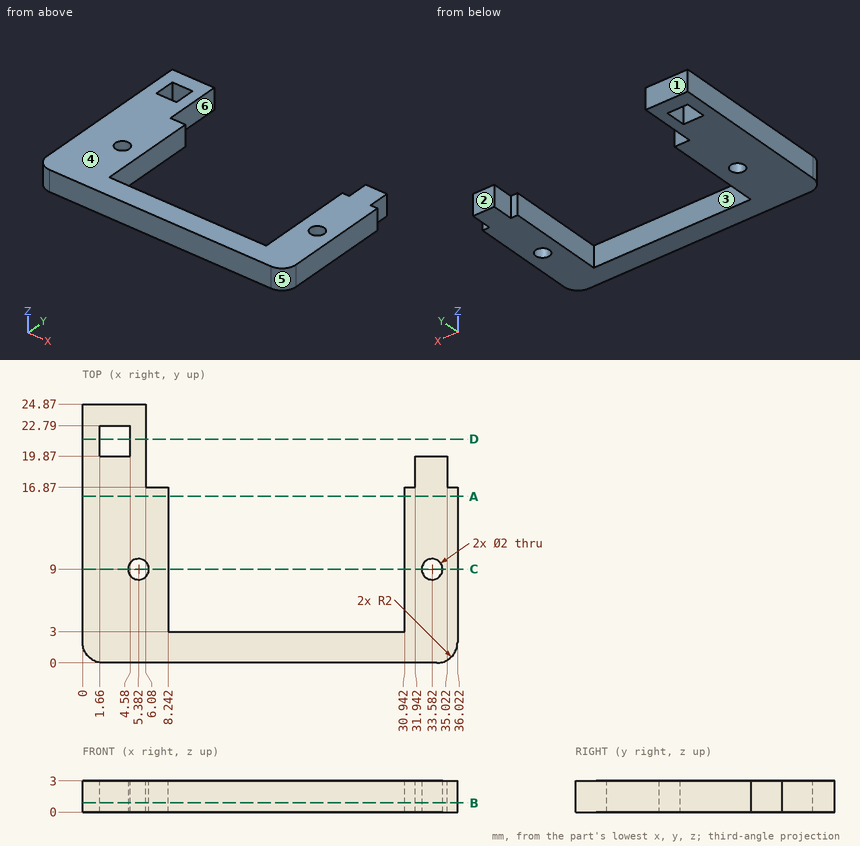
Input: dimensioned drawing with shaded views. Units: mm. Origin: part minimum x, y, z. A direction names the side the tool comes from. Round coordinates to 2 decimals unless told otherwise and drop trailing zeros. Loops run counter-clockwise (first coordinate to the right, second up) from the corner with the lowest first, then second, coordinate; pieces in that order, holes last. Notation, with made-up numbers: (0, 36.25) -> (44, 36.25) arc R13 ccw to (44, 60.25) -> close; hole circle Ø4 at (-24.5, 2.25). An arc over 180 degrees is marked (long way). Answer as a JSON object with one key per item and string values. Group by question number.
1) Section query B-B on z = 0.9. Output: boundary loops of the cut face in (x, y), plus the area to 3 significant figures.
2) Reachability of the marked faces 1, 2 and 3 from +Z, -Z, +X, -X, +Y, -Y: full face, straight path, thin tool, end or side. Return the list, or none.
3) Section query C-C on y = 9. Output: boundary loops of the cut face in (x, z).
4) Section query A-A on y = 16. Output: boundary loops of the cut face in (x, z).
5) Pin query (flat end, axial travel): pin 1 (1.5 mm diameter, centred on y = 20.5, z = 1, fed in from +X); pin 2 (1.5 mm diameter, centred on y = 21, z = 1.5, fed in from +X); pin 3 (0.6 mm diameter, centred on x = 7, z = 1, fed in from +Y). Return the tip coordinate at first contact, or that it passes through.
6) Ray query, L1, parallel to X at y = 14.5, z = 2.4; L2, parallel to Y at x = 5.5, z = 0.1; L3, parallel to X at y = 22, z = 0.2. Return the intervals inside material, ascending.
7) Draft query along X for the marked faces 4, 5 and 6. Return one class per face: +X half, -X half, draft (parallel to the pull), parting line (faces both ways), or undercut.
8) Section query D-D on y = 21.5. Output: boundary loops of the cut face in (x, z).
Reply:
{
 "1": {"outline": "(0, 2) arc R2 ccw to (2, 0) -> (34.02, 0) arc R2 ccw to (36.02, 2) -> (36.02, 16.87) -> (35.02, 16.87) -> (35.02, 19.87) -> (31.94, 19.87) -> (31.94, 16.87) -> (30.94, 16.87) -> (30.94, 3) -> (8.24, 3) -> (8.24, 16.87) -> (6.08, 16.87) -> (6.08, 24.87) -> (0, 24.87) -> close; hole (1.66, 19.87) -> (4.58, 19.87) -> (4.58, 22.79) -> (1.66, 22.79) -> close; hole circle Ø2 at (5.38, 9); hole circle Ø2 at (33.58, 9)", "area": "334 mm2"},
 "2": {"face 1": "+Z, -Z, +X, -X, +Y", "face 2": "+Z, -Z, +X, +Y", "face 3": "+Z, -Z, +Y"},
 "3": {"outline": "(0, 0) -> (4.38, 0) -> (4.38, 3) -> (0, 3) -> close; (6.38, 0) -> (8.24, 0) -> (8.24, 3) -> (6.38, 3) -> close; (30.94, 0) -> (32.58, 0) -> (32.58, 3) -> (30.94, 3) -> close; (34.58, 0) -> (36.02, 0) -> (36.02, 3) -> (34.58, 3) -> close"},
 "4": {"outline": "(0, 0) -> (8.24, 0) -> (8.24, 3) -> (0, 3) -> close; (30.94, 0) -> (36.02, 0) -> (36.02, 3) -> (30.94, 3) -> close"},
 "5": {"pin 1": "stops at x = 35.02", "pin 2": "stops at x = 6.08", "pin 3": "stops at y = 16.87"},
 "6": {"L1": "x = 0 to 8.24, 30.94 to 36.02", "L2": "y = 0 to 8.01, 9.99 to 24.87", "L3": "x = 0 to 1.66, 4.58 to 6.08"},
 "7": {"face 4": "draft", "face 5": "+X half", "face 6": "undercut"},
 "8": {"outline": "(0, 0) -> (1.66, 0) -> (1.66, 3) -> (0, 3) -> close; (4.58, 0) -> (6.08, 0) -> (6.08, 3) -> (4.58, 3) -> close"}
}
